Autodesk Inventor part; units mm, degrees
ref_plane "Work Plane2" through (0, 17.5, 15) normal (0, 0, 1) x (1, 0, 0)
ref_plane "YZ Plane" through (0, 0, 0) normal (1, 0, 0) x (0, 1, 0)
ref_plane "XZ Plane" through (0, 0, 0) normal (0, 1, 0) x (-1, 0, 0)
sketch "Sketch1" plane through (0, 0, 0) normal (0, 0, 1) x (1, 0, 0)
  line L0 (-9, 0) -> (-15, 0)
  line L1 (-15, 0) -> (-15, 35)
  line L2 (-15, 35) -> (-18, 35)
  line L3 (-18, 35) -> (-18, 37)
  line L4 (-18, 37) -> (-16, 39)
  line L5 (-16, 39) -> (-9, 39)
  line L6 (-9, 39) -> (-9, 0)
  line L7 (0, 39) -> (0, 0)
  dimension "d0" = 18
  dimension "d1" = 30
  dimension "d2" = 36
  dimension "d3" = 32
  dimension "d4" = 2
  dimension "d5" = 2
  dimension "d6" = 39
revolve "Revolution1" add sketch "Sketch1" angle 360 about axis through (0, 39, 0) along (0, -1, 0)
chamfer "Chamfer1" distance 1 angle 45 1 edges at (15, 0, 0)
thread "Thread1"
ref_plane "Work Plane2" through (0, 17.5, 15) normal (0, 0, 1) x (1, 0, 0)
sketch "Sketch3" plane through (0, 17.5, 15) normal (0, 0, 1) x (1, 0, 0)
  line L0 (12.5, -7.5) -> (-12.5, -7.5)
  line L1 (-12.5, -7.5) -> (-12.5, 2.5)
  line L2 (-12.5, 2.5) -> (12.5, 2.5)
  line L3 (12.5, 2.5) -> (12.5, -7.5)
  line L4 (12.5, -7.5) -> (-12.5, 2.5) construction
  line L5 (-12.5, -7.5) -> (12.5, 2.5) construction
  point P0 (0, -17.5)
  point P1 (0, -2.5)
  dimension "d16" = 25
  dimension "d17" = 10
  dimension "d18" = 15
extrude "Extrusion1" cut sketch "Sketch3" against normal blind 1.5
Source: CAD feature listing. Evaluate the final solid. Frame: model axes, mm. A direction names the side the tool comes from. Round coordinates to 2 decimals unless told otherwise and drop trailing zeros. Loops run counter-clockwise (first coordinate to the right, second up) from the corner with the lowest first, then second, coordinate; pieces in that order, holes last.
Q1. Access query for faces 1 (the face through (0, 10, 14)), 2 (the face through (4, 35, -15)), 3 (the face through (1.172, 19.227, -8.923)). Directions: +Z, -Z, +X, -X, +Y, -Y. A direction counts if a zero-diameter tool reaches every point of the face in a straight line with its end or side. Return the directions, or none.
Q2. Mould query, pull axis Y, two halves, no side actions, for faces 4 (the face through (2.343, 36.014, 17.847)), 5 (the face through (-9, 0, 3)), 6 (the face through (0, 15, 13.5)), 7 (the face through (3.496, 38.875, 15.742)). Classes: pulls with the +Y half, pulls with the -Y half, needs draft (parallel to the pull), parting line crosses it, or undercut.
Q3. Section C-C, the plane y = 17.5. Return loops of the section in (x, z), plus the area to 3 significant figures.
Q4. First-contact query: P1, Ø1, axis at x = -2, y = 33, coming from the +Z side; P2, Ø8, axis at x = -9, z = 6.5, coming from the -Y side; P3, Ø5, axis at x = -11.5, z = 12.5, coming from the -Y side; P4, Ø1, axis at y = 11.5, z = -4.5, coming from the +X side. Flat tips, straight axial feed; report the tip coordinate or a pass-through.
Q5. Section D-D, the plane y = 33.5. Return loops of the section in (x, z), plus the area to 3 significant figures.
Q6. Section A-A, the plane z = 0. Return loops of the section in (x, y), plus the area to 3 significant figures.
Q7. Section B-B, the plane x = 0. Return loops of the section in (y, z), plus the area to 3 significant figures.
Q8. Ray query, line 1 (Z direction, x = 0, y = 18.5); line 2 (X direction, y = 29, z = 0). Return the intervals inside material, ascending.
Solutions:
1. face 1: +Z, +X, -X
1. face 2: -Y
1. face 3: +Y, -Y
2. face 4: needs draft
2. face 5: pulls with the -Y half
2. face 6: undercut
2. face 7: pulls with the +Y half
3. outline: (-6.54, 13.5) arc R15 ccw (long way) to (6.54, 13.5) - close; hole circle Ø18 at (0, 0)
3. area: 439 mm2
4. P1: stops at z = 14.92
4. P2: stops at y = 0
4. P3: stops at y = 0.49
4. P4: stops at x = 14.46
5. outline: circle Ø30 at (0, 0); hole circle Ø18 at (0, 0)
5. area: 452 mm2
6. outline: (-18, 35) - (-15, 35) - (-15, 1) - (-14, 0) - (-9, 0) - (-9, 39) - (-16, 39) - (-18, 37) - close; (9, 0) - (14, 0) - (15, 1) - (15, 35) - (18, 35) - (18, 37) - (16, 39) - (9, 39) - close
6. area: 487 mm2
7. outline: (0, -14) - (1, -15) - (35, -15) - (35, -18) - (37, -18) - (39, -16) - (39, -9) - (0, -9) - close; (0, 9) - (39, 9) - (39, 16) - (37, 18) - (35, 18) - (35, 15) - (20, 15) - (20, 13.5) - (10, 13.5) - (10, 15) - (1, 15) - (0, 14) - close
7. area: 472 mm2
8. line 1: z = -15 to -9, 9 to 13.5
8. line 2: x = -15 to -9, 9 to 15
